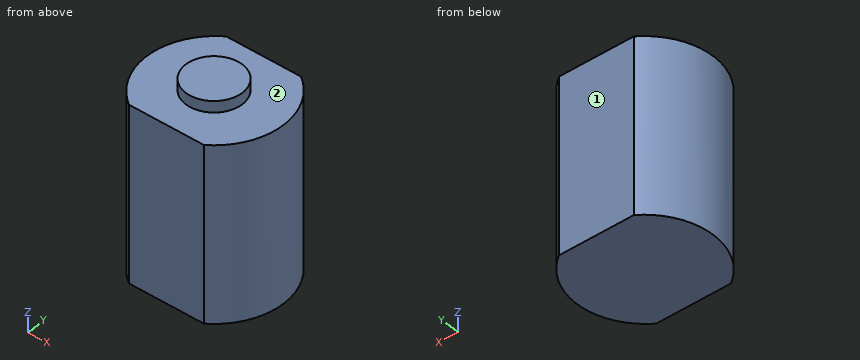
from build123d import *

# Parameters (mm, degrees)
F1_DEPTH = 15.5
F2_R     = 2.5
F3_DEPTH = 1


with BuildPart() as f1:
    # F0 (on Top) → F1 (new body)
    with BuildSketch(Plane.XY):
        with BuildLine():
            ThreePointArc((3.4, -5.05), (6.05, 0), (3.4, 5.05))
            Line((3.4, 5.05), (-3.4, 5.05))
            ThreePointArc((-3.4, 5.05), (-6.05, 0), (-3.4, -5.05))
            Line((-3.4, -5.05), (3.4, -5.05))
        make_face()
    extrude(amount=F1_DEPTH)

    # F2 (on face) → F3 (join)
    with BuildSketch(Plane.XY.offset(15.5)):
        with Locations((-0.086792, 0)):
            Circle(F2_R)
    extrude(amount=F3_DEPTH)


solid = f1.part
Geometry: final body of the model. Coordinates: model frame, mm. Face numbers are marked on the shaded views. A direction names the side the tool comes from. Give positions to 0.01 mm unless a question says otherwise; leave off trailing zeros. Order: outer loops, then holes, each group sorted by start corner. A loop starts at its lowest first (then second) coordinate and runs counter-clockwise, first axis right, second up. Notation, with made-up numbers: (-17.75, 77.5) - (-2.75, 77.5) arc R27 ccw to (-2.75, 107.5) - close; hole circle Ø11 at (24.25, 53). An arc over 180 degrees is marked (long way). Use CSV: the item, a comma, the result in double quotes.
1. Contact query for flat-ended pins moving along their axis: pin 1 (2 mm diameter, centred on y = 2.5, z = 6, fed in from -X); pin 2 (2 mm diameter, centred on y = -1.5, z = 2.5, fed in from -X). Output: stop coordinate, or through.
Answers below:
pin 1,"x = -5.86"
pin 2,"x = -6.03"
2. Section query A-A (y = 0). Output: boundary loops of the cut face in (x, z).
Answers below:
outline,"(-6.05, 0) - (6.05, 0) - (6.05, 15.5) - (2.41, 15.5) - (2.41, 16.5) - (-2.59, 16.5) - (-2.59, 15.5) - (-6.05, 15.5) - close"
3. Section query B-B (x = -1). Output: boundary loops of the cut face in (y, z).
Answers below:
outline,"(-5.05, 0) - (5.05, 0) - (5.05, 15.5) - (2.33, 15.5) - (2.33, 16.5) - (-2.33, 16.5) - (-2.33, 15.5) - (-5.05, 15.5) - close"
4. Material intervals for line 1 along Z through (x, y) = (3, -1.5); line 2 along Y through (x, z) = (-4.75, 10); line 3 along X through (y, z) = (-1.5, 13.25), sorted ascending. Write a range as from..to.
Answers below:
line 1,"0..15.5"
line 2,"-3.78..3.78"
line 3,"-5.86..5.86"
5. Section query C-C (z = 11). Output: boundary loops of the cut face in (x, y), plus the area to 3 significant figures.
Answers below:
outline,"(-3.4, -5.05) - (3.4, -5.05) arc R6.14 ccw to (3.4, 5.05) - (-3.4, 5.05) arc R6.14 ccw to start"
area,"106 mm2"
6. Section query D-D (y = 3.75). Output: boundary loops of the cut face in (x, z).
Answers below:
outline,"(-4.77, 0) - (4.77, 0) - (4.77, 15.5) - (-4.77, 15.5) - close"
7. Access query for the marked faces 1 and 2. Directions: +Z, -Z, +X, -X, +Y, -Y. A direction counts if a zero-diameter tool reaches every point of the face in a straight line with its end or side. Return the directions, or none.
Answers below:
face 1,"+Z, -Z, +X, -X, +Y"
face 2,"+Z"
